from build123d import *

# Parameters (mm, degrees)
SKETCH_2_W      = 1
SKETCH_2_H      = 5
EXTRUDE_1_DEPTH = 1.8
SKETCH_3_W      = 4
SKETCH_3_H      = 6
EXTRUDE_2_DEPTH = 1.5


with BuildPart() as part:
    # 草圖2 → 伸長1 (new body)
    with BuildSketch(Plane.XY):
        Rectangle(SKETCH_2_W, SKETCH_2_H)
    extrude(amount=EXTRUDE_1_DEPTH)

    # 草圖3 → 伸長2 (add)
    with BuildSketch(Plane(origin=(0, 0, 0), x_dir=(-1, 0, 0), z_dir=(0, 0, -1))):
        Rectangle(SKETCH_3_W, SKETCH_3_H)
    extrude_2 = extrude(amount=EXTRUDE_2_DEPTH)

    # 鏡射1: 伸長2 across plane
    add(extrude_2.mirror(Plane.XY.offset(0.9)))

    # 草圖4 → 疊層拉伸1 section 0
    with BuildSketch(Plane(origin=(0, 0, -6.5), x_dir=(-1, 0, 0), z_dir=(0, 0, -1))):
        with BuildLine():
            Line((-1, 2.25), (1, 2.25))
            Line((1, 2.25), (1, -2.25))
            Line((1, -2.25), (-1, -2.25))
            Line((-1, -2.25), (-1, 2.25))
        make_face()
    # 草圖5 → 疊層拉伸1 section 1
    with BuildSketch(Plane(origin=(0, 0, -1.5), x_dir=(-1, 0, 0), z_dir=(0, 0, -1))):
        with BuildLine():
            Line((-1.85, 2.45), (1.85, 2.45))
            Line((1.85, 2.45), (1.85, -2.45))
            Line((1.85, -2.45), (-1.85, -2.45))
            Line((-1.85, -2.45), (-1.85, 2.45))
        make_face()
    loft()


solid = part.part
Work out the finished part from the listing and answer in its coordinate system (mm). A direction names the side the tool comes from. Give positions to 0.01 mm unless a question says otherwise; leave off trailing zeros. Order: outer loops, then holes, each group sorted by start corner. A loop starts at its lowest first (then second) coordinate and runs counter-clockwise, first axis right, second up. Notation, with made-up numbers: (55.25, -7) - (101.25, -7) arc R8 cw to (101.25, 4) - close; hole circle Ø2 at (85.5, 80.5). An arc over 180 degrees is marked (long way). Answer as CSV lines item,"result". Start each with the question number.
Q1. The part is cut by section A-A (z = 1). Write down the section's boundary in (x, y), then the cut area to 3 significant figures.
Q2. Find the intervals of material crossed by L1, parallel to Z at x = -0.55, y = 1.1; L2, parallel to X at y = -1.4, z = 1.5; L3, parallel to X at y = -1.25, z = -5 (3 decimals), in increasing order. Write a range as [from, to].
Q3. Given pin 1 Ø0.5 at (x, z) = (0, 0.5) entering from +Y; pin 2 Ø1.4 at (y, z) = (1, 1) entering from -X; pin 3 Ø0.8 at (x, z) = (0, 1) entering from -Y, each flat-ended and moving along its own axis, determine where each tip first touches the part or whether it passes through.
Q4. For faces 1 (the face through (0.5, 0, 1)), 2 (the face through (-2, 0, 3)), 3 (the face through (0, -2.5, 1)), determine the directions among +Z, -Z, +X, -X, +Y, -Y from which every point of the face is accessible in a straight line to the end or side of a thin tool.
Q5. The mould has two halves that part along Z. Classify faces 4 (the face through (2, 0, 3)), 5 (the face through (0, 0, -6.5)), 6 (the face through (-0.5, 0, 1)), 7 (the face through (0, 2.5, 1)): +Z half, -Z half, draft (parallel to the pull), parting line (faces both ways), or undercut.
Check result:
1,outline,"(-0.5, -2.5) - (0.5, -2.5) - (0.5, 2.5) - (-0.5, 2.5) - close"
1,area,"5.00 mm²"
2,L1,"z = [-6.5, 0], [1.8, 3.3]"
2,L2,"x = [-0.5, 0.5]"
2,L3,"x = [-1.255, 1.255]"
3,pin 1,"stops at y = 2.5"
3,pin 2,"stops at x = -0.5"
3,pin 3,"stops at y = -2.5"
4,face 1,"+X, +Y, -Y"
4,face 2,"+Z, -Z, -X, +Y, -Y"
4,face 3,"+X, -X, -Y"
5,face 4,"draft"
5,face 5,"-Z half"
5,face 6,"undercut"
5,face 7,"undercut"
